Work out the finished part from the listing and answer in its coordinate system (mm). A direction names the side the tool comes from. Round coordinates to 2 decimals unless told otherwise and drop trailing zeros. Loops run counter-clockwise (first coordinate to the right, second up) from the corner with the lowest first, then second, coordinate; pieces in that order, holes last.
from build123d import *

# Parameters (mm, degrees)
Y_KSEKLIK_EKSTR_ZYON2_DEPTH             = 62.5
KES_EKSTR_ZYON5_DEPTH                   = 15
KES_EKSTR_ZYON6_DEPTH                   = 15
M3_BO_LUKLU_DELIK1_D                    = 3.2
M3_BO_LUKLU_DELIK1_DEPTH                = 11.5
M3_BO_LUKLU_DELIK1_TIP                  = 0.9613769904440965
M3X0_5_HELISARMAL_IN_DI_LI_DELIK2_D     = 3.15
M3X0_5_HELISARMAL_IN_DI_LI_DELIK2_DEPTH = 11
M3X0_5_HELISARMAL_IN_DI_LI_DELIK2_TIP   = 0.9463554749684074
RADYUS1_R                               = 1
Y_KSEKLIK_EKSTR_ZYON3_DEPTH             = 10
M3X0_5_HELISARMAL_IN_DI_LI_DELIK1_D     = 3.15
M3X0_5_HELISARMAL_IN_DI_LI_DELIK1_DEPTH = 10
M3X0_5_HELISARMAL_IN_DI_LI_DELIK1_TIP   = 0.9463554749684074
DAIRESEL_KAPLAMA1_COUNT                 = 2
DAIRESEL_KAPLAMA1_ANGLE                 = 180.0000000000004


with BuildPart() as part:
    # Çizim1 → Yükseklik-Ekstrüzyon2 (new, symmetric)
    with BuildSketch(Plane.XY):
        with BuildLine():
            Line((32.04001404494075, 45), (-32.04001404494075, 45))
            ThreePointArc((-32.04001404494075, 45), (-33.696486936063444, 44.7176368619231), (-35.165869073715456, 43.90243902439025))
            ThreePointArc((-35.165869073715456, 43.90243902439025), (-55.65852190175254, 8.135812172864675), (-46.260809547607366, -32))
            Line((-46.260809547607366, -32), (-35.06245411157585, -32))
            Line((-35.06245411157585, -32), (-35.06245411157585, -28))
            Line((-35.06245411157585, -28), (-45.2941773299836, -28.000000000000007))
            ThreePointArc((-45.2941773299836, -28.000000000000007), (-52.56891292419714, 8.48951670992989), (-34.1779294904093, 40.83419689119171))
            ThreePointArc((-34.1779294904093, 40.83419689119171), (-32.67592718411632, 41.69952042531781), (-30.968734233093876, 41.99999999999999))
            Line((-30.968734233093876, 41.99999999999999), (30.968734233093905, 41.99999999999997))
            ThreePointArc((30.968734233093905, 41.99999999999997), (32.675927184116354, 41.699520425317786), (34.17792949040933, 40.83419689119169))
            ThreePointArc((34.17792949040933, 40.83419689119169), (52.56891292419713, 8.489516709929875), (45.2941773299836, -27.99999999999998))
            Line((45.2941773299836, -27.99999999999998), (35.06245411157585, -27.99999999999998))
            Line((35.06245411157585, -27.99999999999998), (35.06245411157587, -31.999999999999957))
            Line((35.06245411157587, -31.999999999999957), (46.260809547607366, -32))
            ThreePointArc((46.260809547607366, -32), (55.65852190175254, 8.13581217286468), (35.165869073715456, 43.90243902439025))
            ThreePointArc((35.165869073715456, 43.90243902439025), (33.696486936063444, 44.7176368619231), (32.04001404494075, 45))
        make_face()
    extrude(amount=Y_KSEKLIK_EKSTR_ZYON2_DEPTH, both=True)

    # Çizim3 → Kes-Ekstrüzyon5 (cut)
    with BuildSketch(Plane.XY.offset(62.5)):
        with BuildLine():
            Line((-42.56245411157586, -31.99999999999998), (-42.56245411157586, -32.283572214894534))
            Line((-42.56245411157586, -32.283572214894534), (-35.06245411157585, -32.283572214894534))
            Line((-35.06245411157585, -32.283572214894534), (-35.06245411157585, -32))
            Line((-35.06245411157585, -32), (-35.06245411157585, -28))
            Line((-35.06245411157585, -28), (-45.2941773299836, -28.000000000000007))
            ThreePointArc((-45.2941773299836, -28.000000000000007), (-43.97382087179262, -30.031076869394756), (-42.56245411157586, -31.99999999999998))
        make_face()
        with BuildLine():
            Line((35.06245411157585, -27.99999999999998), (45.294177329983604, -27.99999999999998))
            ThreePointArc((45.294177329983604, -27.99999999999998), (43.97389225931995, -30.030972337999984), (42.56260624715447, -31.999797647011572))
            Line((42.56260624715447, -31.999797647011572), (42.56260624715447, -32.40361379134536))
            Line((42.56260624715447, -32.40361379134536), (35.06245411157587, -32.40361379134536))
            Line((35.06245411157587, -32.40361379134536), (35.06245411157587, -31.999999999999957))
            Line((35.06245411157587, -31.999999999999957), (35.06245411157585, -27.99999999999998))
        make_face()
    extrude(amount=-KES_EKSTR_ZYON5_DEPTH, mode=Mode.SUBTRACT)

    # Çizim4 → Kes-Ekstrüzyon6 (cut)
    with BuildSketch(Plane(origin=(0, 45, 0), x_dir=(1, 0, 0), z_dir=(0, 1, 0))):
        Polygon((23.75, 62.49999999999993), (-23.75, 62.5), (-23.749999999999993, 4.499999999999997), (23.749999999999993, 4.499999999999997), align=None)
    extrude(amount=-KES_EKSTR_ZYON6_DEPTH, mode=Mode.SUBTRACT)

    # M3 Boşluklu Delik1
    with Locations(Plane(origin=(0, 45, 0), x_dir=(1, 0, 0), z_dir=(0, 1, 0))):
        with Locations((0, -2.45), (-28.75, 42.5), (28.75, 42.5)):
            Hole(M3_BO_LUKLU_DELIK1_D / 2, depth=M3_BO_LUKLU_DELIK1_DEPTH)
            with Locations((0, 0, -(M3_BO_LUKLU_DELIK1_DEPTH + M3_BO_LUKLU_DELIK1_TIP / 2))):  # 118° drill point
                Cone(0, M3_BO_LUKLU_DELIK1_D / 2, M3_BO_LUKLU_DELIK1_TIP, mode=Mode.SUBTRACT)

    # M3x0.5 Helisarmal İçin Dişli Delik2
    with Locations(Plane.XZ.offset(32)):
        with Locations((41.000809548, -27.5), (-41.000809548, -27.5), (-41.000809548, 27.5), (41.000809548, 27.5)):
            Hole(M3X0_5_HELISARMAL_IN_DI_LI_DELIK2_D / 2, depth=M3X0_5_HELISARMAL_IN_DI_LI_DELIK2_DEPTH)
            with Locations((0, 0, -(M3X0_5_HELISARMAL_IN_DI_LI_DELIK2_DEPTH + M3X0_5_HELISARMAL_IN_DI_LI_DELIK2_TIP / 2))):  # 118° drill point
                Cone(0, M3X0_5_HELISARMAL_IN_DI_LI_DELIK2_D / 2, M3X0_5_HELISARMAL_IN_DI_LI_DELIK2_TIP, mode=Mode.SUBTRACT)

    # Radyus1
    radyus1_edges = [part.edges().sort_by_distance(p)[0] for p in [
        (35.06245411157585, -27.99999999999998, -7.5),
        (-35.06245411157585, -28, -7.5),
    ]]
    fillet(radyus1_edges, radius=RADYUS1_R)

    # Çizim14 → Yükseklik-Ekstrüzyon3 (add)
    with BuildSketch(Plane(origin=(0, 0, -62.5), x_dir=(-1, 0, 0), z_dir=(0, 0, -1))):
        with BuildLine():
            Line((36.06245411157586, -23), (42.41535688874963, -23.000000000000004))
            ThreePointArc((42.41535688874963, -23.000000000000004), (47.39521291696829, 9.04191863241662), (30.968734233093883, 37))
            Line((30.968734233093883, 37), (23.75000000000001, 36.999999999999986))
            Line((23.75000000000001, 36.999999999999986), (23.749999999999996, 42.999999999999986))
            Line((23.749999999999996, 42.999999999999986), (30.968734233093873, 43))
            ThreePointArc((30.968734233093873, 43), (33.0173657743208, 42.63942451038137), (34.81976854187237, 41.60103626943006))
            ThreePointArc((34.81976854187237, 41.60103626943006), (53.59999153018334, 8.372777792601147), (45.848255146733784, -29.000000000000004))
            Line((45.848255146733784, -29.000000000000004), (36.06245411157585, -29))
            Line((36.06245411157585, -29), (36.06245411157586, -23))
        make_face()
        with BuildLine():
            Line((-23.75, 42.999999999999986), (-30.968734233093905, 42.99999999999998))
            ThreePointArc((-30.968734233093905, 42.99999999999998), (-33.01736577432084, 42.639424510381346), (-34.819768541872406, 41.601036269430026))
            ThreePointArc((-34.819768541872406, 41.601036269430026), (-53.59999153018334, 8.372777792601134), (-45.8482551467338, -28.999999999999982))
            Line((-45.8482551467338, -28.999999999999982), (-36.06245411157586, -28.999999999999982))
            Line((-36.06245411157586, -28.999999999999982), (-36.06245411157586, -22.99999999999998))
            Line((-36.06245411157586, -22.99999999999998), (-42.415356888749635, -22.99999999999998))
            ThreePointArc((-42.415356888749635, -22.99999999999998), (-47.39521291696828, 9.041918632416632), (-30.968734233093908, 36.99999999999998))
            Line((-30.968734233093908, 36.99999999999998), (-23.749999999999996, 36.999999999999986))
            Line((-23.749999999999996, 36.999999999999986), (-23.75, 42.999999999999986))
        make_face()
    extrude(amount=-Y_KSEKLIK_EKSTR_ZYON3_DEPTH)

    # M3x0.5 Helisarmal İçin Dişli Delik1
    with Locations(Plane(origin=(0, 0, -62.5), x_dir=(-1, 0, 0), z_dir=(0, 0, -1))):
        with Locations((36.769552622, 36.769552622), (-52, 0), (-36.769552622, 36.769552622), (-45.033320997, -26), (52, 0), (45.033320997, -26)):
            Hole(M3X0_5_HELISARMAL_IN_DI_LI_DELIK1_D / 2, depth=M3X0_5_HELISARMAL_IN_DI_LI_DELIK1_DEPTH)
            with Locations((0, 0, -(M3X0_5_HELISARMAL_IN_DI_LI_DELIK1_DEPTH + M3X0_5_HELISARMAL_IN_DI_LI_DELIK1_TIP / 2))):  # 118° drill point
                Cone(0, M3X0_5_HELISARMAL_IN_DI_LI_DELIK1_D / 2, M3X0_5_HELISARMAL_IN_DI_LI_DELIK1_TIP, mode=Mode.SUBTRACT)

    # Çizim22 → M3 Altıgen Alyan Havşa Başlı Kör Vida İçin Havşa3 (revolve, cut)
    with BuildSketch(Plane(origin=(56.25, -7e-17, 55), x_dir=(0, 0, -1), z_dir=(0, 1, 0))):
        Polygon((0, 0), (-1.4e-15, 9.961376990444082), (1.5999999999999868, 8.999999999999995), (1.5999999999999885, 1.7600000000000116), (3.3600000000000003, -1.73e-15), align=None)
    m3_alt_gen_alyan_hav_a_ba_l_k_r_vida_i = revolve(axis=Axis((62.599999999999994, -7e-17, 55), (-1, 0, 0)), mode=Mode.SUBTRACT)

    # Dairesel Kaplama1: M3 Altıgen Alyan Havşa Başlı Kör Vida İçin Havşa3 ×2 about axis
    dairesel_kaplama1_axis = Axis((0, 0, 62.5), (0, 0, 1))
    for i in range(1, DAIRESEL_KAPLAMA1_COUNT):
        add(m3_alt_gen_alyan_hav_a_ba_l_k_r_vida_i.rotate(dairesel_kaplama1_axis, i * DAIRESEL_KAPLAMA1_ANGLE / (DAIRESEL_KAPLAMA1_COUNT - 1)), mode=Mode.SUBTRACT)


solid = part.part
Item 1: For faces 5 (the face through (-41.728, -29.972, -28.897)), 6 (the face through (32.65, 41.71, 5.8)), 7 (the face through (-36.062, -26, -58)), 8 (the face through (-48, 10, -52.5)), determine the directions among +Z, -Z, +X, -X, +Y, -Y from which every point of the face is accessible in a straight line to the end or side of a thin tool.
Item 2: Determine the mould class of faces 1 (the face through (40.274, -29.972, -28.897)), 2 (the face through (-47.48, 8.59, -57.57)), 3 (the face through (-39, -23, -58)), 4 (the face through (-41, -32, 1)) for opening direction Y: pulls with the +Y half, pulls with the -Y half, needs draft (parallel to the pull), parting line crosses it, or undercut.
Item 3: Section A-A, the plane z = 27.5 is taken. Give the vertices of the cut face in (x, y), plus the area to 3 significant figures.
Item 4: Section D-D, the plane y = -10.5 is taken. Give the vertices of the cut face in (x, z).
Item 5: Section B-B, the plane x = -28.75 is taken. Give the vertices of the cut face in (y, z).
Item 6: Straight lines are drawn through the part: line 1 (Z direction, x = -28.75, y = 43); line 2 (Z direction, x = -53.95, y = 0); line 3 (X direction, y = 35.5, z = 20). For each, find the intervals that lie inside material, in ascending order.
Item 7: Section C-C, the plane z = -38.5 is taken. Give the vertices of the cut face in (x, y).
Item 8: Each of these flat-tipped pins is pushed along its axis until it touches: P1, Ø5, axis at y = -8, z = 49.5, coming from the +X side; P2, Ø5, axis at y = 24, z = -45.5, coming from the -X side; P3, Ø2, axis at y = 20.5, z = -47, coming from the +X side. Where does it stop, or does it pass through?
Answer below:
1. face 5: -Y
1. face 6: +Z, -Y
1. face 7: +Z, -Z
1. face 8: +Z
2. face 1: needs draft
2. face 2: undercut
2. face 3: undercut
2. face 4: pulls with the -Y half
3. outline: (-46.26, -32) - (-42.58, -32) - (-42.58, -28) - (-45.29, -28) arc R53.25 cw to (-34.18, 40.83) arc R5 cw to (-30.97, 42) - (30.97, 42) arc R5 cw to (34.18, 40.83) arc R53.25 cw to (45.29, -28) - (42.58, -28) - (42.58, -32) - (46.26, -32) arc R56.25 ccw to (35.17, 43.9) arc R5 ccw to (32.04, 45) - (-32.04, 45) arc R5 ccw to (-35.17, 43.9) arc R56.25 ccw to start; (-39.43, -32) - (-35.06, -32) - (-35.06, -29) arc R1 ccw to (-36.06, -28) - (-39.43, -28) - close; (35.06, -32) - (39.43, -32) - (39.43, -28) - (36.06, -28) arc R1 ccw to (35.06, -29) - close
3. area: 752 mm2
4. outline: (-55.26, -62.5) - (-47.09, -62.5) - (-47.09, -52.5) - (-52.2, -52.5) - (-52.2, 62.5) - (-55.26, 62.5) - close; (47.09, -62.5) - (55.26, -62.5) - (55.26, 62.5) - (52.2, 62.5) - (52.2, -52.5) - (47.09, -52.5) - close
5. outline: (37, -62.5) - (45, -62.5) - (45, -44.1) - (42, -44.1) - (42, -52.5) - (37, -52.5) - close; (42, -40.9) - (45, -40.9) - (45, 62.5) - (42, 62.5) - close
6. line 1: z = -62.5 to -44.1, -40.9 to 62.5
6. line 2: z = -62.5 to 53.4, 56.6 to 62.5
6. line 3: x = -43.63 to -39.69, 39.69 to 43.63
7. outline: (-46.26, -32) - (-35.06, -32) - (-35.06, -29) arc R1 ccw to (-36.06, -28) - (-45.29, -28) arc R53.25 cw to (-34.18, 40.83) arc R5 cw to (-30.97, 42) - (-23.75, 42) - (-23.75, 45) - (-32.04, 45) arc R5 ccw to (-35.17, 43.9) arc R56.25 ccw to start; (23.75, 42) - (30.97, 42) arc R5 cw to (34.18, 40.83) arc R53.25 cw to (45.29, -28) - (36.06, -28) arc R1 ccw to (35.06, -29) - (35.06, -32) - (46.26, -32) arc R56.25 ccw to (35.17, 43.9) arc R5 ccw to (32.04, 45) - (23.75, 45) - close
8. P1: stops at x = 55.98
8. P2: stops at x = -51.98
8. P3: stops at x = 52.76
